Autodesk Inventor part; units mm, degrees
ref_plane "YZ Plane" through (0, 0, 0) normal (1, 0, 0) x (0, 1, 0)
ref_plane "XZ Plane" through (0, 0, 0) normal (0, 1, 0) x (-1, 0, 0)
ref_plane "XY Plane" through (0, 0, 0) normal (0, 0, 1) x (1, 0, 0)
sketch "Boceto1" plane through (0, 0, 0) normal (0, 1, 0) x (-1, 0, 0)
  circle A0 centre (37, 37) radius 4.15
  line L0 (25, -33.5) -> (25, -49)
  line L1 (25, -49) -> (49, -49)
  line L2 (49, -49) -> (49, -25)
  line L3 (49, -25) -> (33.5, -25)
  line L4 (33.5, -25) -> (33.5, 25)
  line L5 (33.5, 25) -> (49, 25)
  line L6 (49, 25) -> (49, 49)
  line L7 (49, 49) -> (25, 49)
  line L8 (25, 49) -> (25, 33.5)
  line L9 (25, 33.5) -> (-25, 33.5)
  line L10 (-25, 33.5) -> (-25, 49)
  line L11 (-25, 49) -> (-49, 49)
  line L12 (-49, 49) -> (-49, 25)
  line L13 (-49, 25) -> (-33.5, 25)
  line L14 (-33.5, 25) -> (-33.5, -25)
  line L15 (-33.5, -25) -> (-49, -25)
  line L16 (-49, -25) -> (-49, -49)
  line L17 (-49, -49) -> (-25, -49)
  line L18 (-25, -49) -> (-25, -33.5)
  line L19 (-25, -33.5) -> (25, -33.5)
  circle A1 centre (0, 0) radius 5 construction
  line L20 (49, -49) -> (-49, -49) construction
  line L21 (-49, -49) -> (-49, 49)
  line L22 (-49, 49) -> (49, 49) construction
  line L23 (49, 49) -> (49, -49) construction
  line L24 (49, -49) -> (25.0011, -49) construction
  line L25 (25.0011, -49) -> (25.0011, -25) construction
  line L26 (49, -25) -> (49, -49) construction
  line L27 (0, -49) -> (0, 49) construction
  line L28 (49, 0) -> (-49, 0) construction
  line L29 (49, 49) -> (25, 49) construction
  line L30 (25, 49) -> (25, 25) construction
  line L31 (25, 25) -> (49, 25) construction
  line L32 (49, 25) -> (49, 49) construction
  line L33 (49, 49) -> (25, 25) construction
  line L34 (49, 25) -> (25, 49) construction
  circle A2 centre (-37, 37) radius 4.15
  circle A3 centre (-37, -37) radius 4.15
  circle A4 centre (37, -37) radius 4.15
  line L35 (29.5, 29.5) -> (-29.5, 29.5)
  line L36 (-29.5, 29.5) -> (-29.5, -29.5)
  line L37 (-29.5, -29.5) -> (29.5, -29.5)
  line L38 (29.5, -29.5) -> (29.5, 29.5)
  line L39 (29.5, 29.5) -> (-29.5, -29.5) construction
  line L40 (-29.5, 29.5) -> (29.5, -29.5) construction
  circle A5 centre (0, 0) radius 2.5 construction
  point P0 (33.5, 0)
  point P1 (0, -33.5)
  point P2 (0, 33.5)
  point P3 (-33.5, 0)
  dimension "d0" = 33.5
  dimension "d1" = 33.5
  dimension "d4" = 8.3
  dimension "d6" = 49
  dimension "d7" = 49
  dimension "d8" = 98
  dimension "d9" = 98
  dimension "d10" = 15.5
  dimension "d11" = 15.5
  dimension "d12" = 15.5
  dimension "d13" = 15.5
  dimension "d14" = 50
  dimension "d15" = 50
  dimension "d16" = 15.5
  dimension "d17" = 15.5
  dimension "d18" = 15.5
  dimension "d19" = 50
  dimension "d20" = 25
  dimension "d21" = 25
  dimension "d22" = 25
  dimension "d23" = 25
  dimension "d24" = 10
  dimension "d26" = 8.5
  dimension "d27" = 8.5
  dimension "d28" = 24
  dimension "d29" = 15.5
  dimension "d30" = 24
  dimension "d31" = 8.5
  dimension "d32" = 24
  dimension "d33" = 24
  dimension "d36" = 360
  dimension "d41" = 4
  dimension "d46" = 5
  dimension "d49" = 4
extrude "Extrusión1" add sketch "Boceto1" along normal blind 40 contours L19 L18 L17 L16 L15 L14 L13 L12 L11 L10 L9 L8 L7 L6 L5 L4 L3 L2 L1 L0
extrude "Extrusión2" add sketch "Boceto1" along normal blind 6.5 contours L38 L37 L36 L35
sketch "Boceto2" plane through (0, 40, 0) normal (0, 1, 0) x (1, 0, 0)
  line L0 (33.5, -25) -> (33.5, 25)
  line L1 (-33.5, 17.5) -> (33.5, 17.5)
  line L2 (33.5, 17.5) -> (33.5, -17.5)
  line L3 (33.5, -17.5) -> (-33.5, -17.5)
  line L4 (-33.5, -17.5) -> (-33.5, 17.5)
  line L5 (-33.5, 17.5) -> (33.5, -17.5) construction
  line L6 (33.5, 17.5) -> (-33.5, -17.5) construction
  line L7 (17.5, 33.5) -> (-17.5, 33.5)
  line L8 (-17.5, 33.5) -> (-17.5, -33.5)
  line L9 (-17.5, -33.5) -> (17.5, -33.5)
  line L10 (17.5, -33.5) -> (17.5, 33.5)
  line L11 (17.5, 33.5) -> (-17.5, -33.5) construction
  line L12 (-17.5, 33.5) -> (17.5, -33.5) construction
  line L13 (-25, -33.5) -> (25, -33.5)
  line L14 (29.5, 29.5) -> (29.5, -29.5)
  line L15 (-29.5, 29.5) -> (29.5, 29.5)
  line L16 (-29.5, -29.5) -> (-29.5, 29.5)
  line L17 (29.5, -29.5) -> (-29.5, -29.5)
  point P0 (0, 0)
  point P1 (0, 0)
  point P2 (-17.5, 29.5)
  point P3 (17.5, 29.5)
  point P4 (-29.5, -17.5)
  point P5 (-29.5, 17.5)
  point P6 (17.5, -29.5)
  point P7 (-17.5, -29.5)
  point P8 (29.5, 17.5)
  point P9 (29.5, -17.5)
  dimension "d50" = 35
  dimension "d51" = 35
extrude "Extrusión5" cut sketch "Boceto2" against normal up to surface (33.5 mm away) contours L3 L14 L1 L0 | L10 L9 L8 L17 | L15 L8 L7 L10 | L3 L4 L1 L16
fillet "Empalme1" radius 4 12 edges at (49, 20, 49) (49, 20, -49) (49, 20, 25) (25, 20, -49) (-25, 20, -49) (-49, 20, -49) (-49, 20, -25) (-49, 20, 25) (-49, 20, 49) (-25, 20, 49) (25, 20, 49) (49, 20, -25)
chamfer "Chaflán1" distance 3 angle 45 8 edges at (33.5, 20, 25) (33.5, 20, -25) (25, 20, -33.5) (-25, 20, -33.5) (-33.5, 20, -25) (-33.5, 20, 25) (-25, 20, 33.5) (25, 20, 33.5)
sketch "Boceto3" plane through (0, 6.5, 0) normal (0, 1, 0) x (1, 0, 0)
  line L0 (-29.5, -29.5) -> (-29.5, -17.5) construction
  line L1 (29.5, 29.5) -> (29.5, 17.5) construction
  line L2 (-29.5, -29.5) -> (29.5, -29.5)
  line L3 (29.5, -29.5) -> (29.5, 29.5)
  line L4 (29.5, 29.5) -> (-29.5, 29.5)
  line L5 (-29.5, 29.5) -> (-29.5, -29.5)
  line L6 (-29.5, -29.5) -> (-24.5, -29.5) construction
  line L7 (-24.5, -29.5) -> (-24.5, -24.5) construction
  line L8 (-24.5, -24.5) -> (-29.5, -24.5) construction
  line L9 (-29.5, -24.5) -> (-29.5, -29.5) construction
  line L10 (-29.5, 29.5) -> (-24.5, 29.5) construction
  line L11 (-24.5, 29.5) -> (-24.5, 24.5) construction
  line L12 (-24.5, 24.5) -> (-29.5, 24.5) construction
  line L13 (-29.5, 24.5) -> (-29.5, 29.5) construction
  line L14 (29.5, 29.5) -> (24.5, 29.5) construction
  line L15 (24.5, 29.5) -> (24.5, 24.5) construction
  line L16 (24.5, 24.5) -> (29.5, 24.5) construction
  line L17 (29.5, 24.5) -> (29.5, 29.5) construction
  line L18 (29.5, -29.5) -> (24.5, -29.5) construction
  line L19 (24.5, -29.5) -> (24.5, -24.5) construction
  line L20 (24.5, -24.5) -> (29.5, -24.5) construction
  line L21 (29.5, -24.5) -> (29.5, -29.5) construction
  circle A0 centre (24.5, -24.5) radius 2.25
  circle A1 centre (24.5, 24.5) radius 2.25
  circle A2 centre (-24.5, 24.5) radius 2.25
  circle A3 centre (-24.5, -24.5) radius 2.25
  point P0 (0, 0)
  dimension "d61" = 5
  dimension "d62" = 5
  dimension "d63" = 5
  dimension "d64" = 5
  dimension "d65" = 5
  dimension "d66" = 5
  dimension "d67" = 5
  dimension "d68" = 5
  dimension "d69" = 4.5
  dimension "d70" = 4.5
  dimension "d71" = 4.5
  dimension "d72" = 4.5
extrude "Extrusión6" cut sketch "Boceto3" against normal blind 5 contours A0 | A1 | A2 | A3
properties part number "Electronica_3DPrint"
Check sheet for the modelled part. Datum: model origin and axes. Units: mm. A direction names the side the tool comes from. Round coordinates to 2 decimals unless told otherwise and drop trailing zeros. Loops run counter-clockwise (first coordinate to the right, second up) from the corner with the lowest first, then second, coordinate; pieces in that order, holes last. Notation, with made-up numbers: M 25.25,-16.5 L 32.25,-16.5 A6 ccw 32.25,-12.5 Z; hole C 14,78.25 d4. An arc over 180 degrees is marked long. One line per question, with ' | ' between items. Start each with the question number.
Item 1: Gauge pin test, flat ends, axial feed: pin 1 Ø7 at (x, z) = (24.5, 24.5) entering from +Y; pin 2 Ø2 at (x, z) = (24, -25) entering from +Y; pin 3 Ø8 at (x, y) = (17.5, 35.5) entering from +Z. Record the tip position at first contact, or that the pin passes through.
Item 2: Release check for a two-part mould opening along X. For faces 5 (the face through (23.5, 20.3, -35)), 6 (the face through (-35, 19.7, -23.5)), 7 (the face through (-37, 20, -49)) record: released by +X, released by -X, zero draft, split by the parting line, or undercut.
Item 3: Section check A-A (y = 15). State how many separate pieces and enclosed holes the cut face has, and give its area (3 significant figures).
Item 4: Section check B-B (z = -38.5). Record the boundary of the cut face in (x, y), and give its area (3 significant figures).
Item 5: Set-up check for faces 1 (the face through (-31, 23, 17.5)), 2 (the face through (33.5, 6, 0)), 3 (the face through (-29.5, 23, 23)), 4 (the face through (-25, 20, 41)): record each of +Z, -Z, +X, -X, +Y, -Y from which the full face is reachable in a straight line by a thin tool's end or side.
Item 6: Scan lines: probe 1 along Z at (x, y) = (-37, 12); probe 2 along X at (y, z) = (18, -20); probe 3 along X at (y, z) = (16, 36). Record each from-to range of solid material in increasing order.
Item 7: Section check C-C (x = -38.5). Record the boundary of the cut face in (y, z), and give its area (3 significant figures).
Worked out:
1) pin 1: y = 6.5 | pin 2: y = 1.5 | pin 3: z = 33.5
2) face 5: undercut | face 6: released by -X | face 7: zero draft
3) separate pieces: 4 | enclosed holes: 4 | area: 2,240 mm^2
4) outline: M -49,0 L -40.87,0 L -40.87,40 L -49,40 Z; M -33.13,0 L -25,0 L -25,40 L -33.13,40 Z; M 25,0 L 33.13,0 L 33.13,40 L 25,40 Z; M 40.87,0 L 49,0 L 49,40 L 40.87,40 Z | area: 1,300 mm^2
5) face 1: +X, -X, +Y | face 2: +X, +Y, -Y | face 3: +Y | face 4: +Z, +Y, -Y
6) probe 1: -49 to -41.15, -32.85 to -25, 25 to 32.85, 41.15 to 49 | probe 2: -33.5 to -29.5, 29.5 to 33.5 | probe 3: -49 to -41.03, -32.97 to -24.5, 24.5 to 32.97, 41.03 to 49
7) outline: M 0,-49 L 40,-49 L 40,-40.87 L 0,-40.87 Z; M 0,-33.13 L 40,-33.13 L 40,-25 L 0,-25 Z; M 0,25 L 40,25 L 40,33.13 L 0,33.13 Z; M 0,40.87 L 40,40.87 L 40,49 L 0,49 Z | area: 1,300 mm^2
